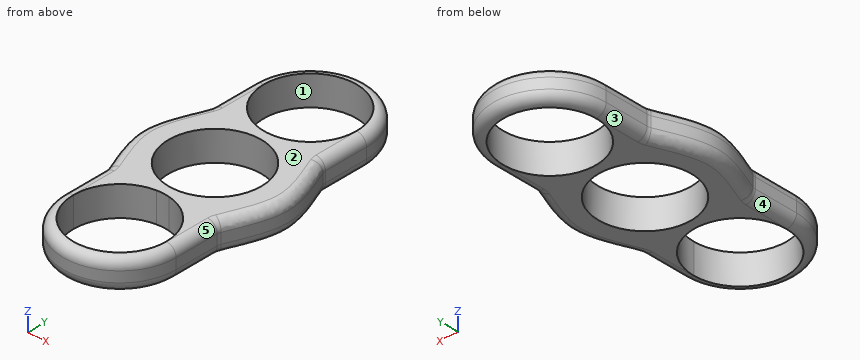
```python
from build123d import *

# Parameters (mm, degrees)
F0_R     = 11.1
F1_DEPTH = 7.1
F2_R     = 2.3


with BuildPart() as f1:
    # F0 (on Top) → F1 (new body)
    with BuildSketch(Plane.XY):
        with BuildLine():
            Line((11.1, 24.4949632536), (13.5, 24.4949632536))
            ThreePointArc((13.5, 24.4949632536), (0, 37.9949632536), (-13.5, 24.4949632536))
            Line((-13.5, 24.4949632536), (-11.1, 24.4949632536))
            ThreePointArc((-11.1, 24.4949632536), (0, 35.5949632536), (11.1, 24.4949632536))
        make_face()
        with BuildLine():
            Line((-13.5, 13.5), (-1.5234116489, 13.5))
            ThreePointArc((-1.5234116489, 13.5), (-8.3701812795, 17.2045541191), (-11.1, 24.4949632536))
            Line((-11.1, 24.4949632536), (-13.5, 24.4949632536))
            Line((-13.5, 24.4949632536), (-13.5, 13.5))
        make_face()
        with BuildLine():
            Line((1.5234116489, 13.5), (13.5, 13.5))
            Line((13.5, 13.5), (13.5, 24.4949632536))
            Line((13.5, 24.4949632536), (11.1, 24.4949632536))
            ThreePointArc((11.1, 24.4949632536), (8.3701812795, 17.2045541191), (1.5234116489, 13.5))
        make_face()
        with BuildLine():
            Line((13.5, -13.5), (13.5, 13.5))
            Line((13.5, 13.5), (1.5234116489, 13.5))
            ThreePointArc((1.5234116489, 13.5), (0, 13.3949632536), (-1.5234116489, 13.5))
            Line((-1.5234116489, 13.5), (-13.5, 13.5))
            Line((-13.5, 13.5), (-13.5, -13.5))
            Line((-13.5, -13.5), (-1.5048250316, -13.5))
            ThreePointArc((-1.5048250316, -13.5), (0, -13.3975225221), (1.5048250316, -13.5))
            Line((1.5048250316, -13.5), (13.5, -13.5))
        make_face()
        Circle(F0_R, mode=Mode.SUBTRACT)
        with BuildLine():
            add(Edge.make_bspline(
                [(13.5, 13.5), (15.2430341691, 9), (19.7569658309, 0), (15.2430341691, -9), (13.5, -13.5)],
                knots=[0, 0, 0, 0, 0.5, 1, 1, 1, 1], degree=3))
            Line((13.5, 13.5), (13.5, -13.5))
        make_face()
        with BuildLine():
            Line((-13.5, -13.5), (-13.5, 13.5))
            add(Edge.make_bspline(
                [(-13.5, 13.5), (-15.2435445338, 9), (-19.7564554662, 0), (-15.2435445338, -9), (-13.5, -13.5)],
                knots=[0, 0, 0, 0, 0.5, 1, 1, 1, 1], degree=3))
        make_face()
        with BuildLine():
            ThreePointArc((-11.1, -24.4975225221), (-8.3640169133, -17.2000420614), (-1.5048250316, -13.5))
            Line((-1.5048250316, -13.5), (-13.5, -13.5))
            Line((-13.5, -13.5), (-13.5, -24.4975225221))
            Line((-13.5, -24.4975225221), (-11.1, -24.4975225221))
        make_face()
        with BuildLine():
            Line((13.5, -24.4975225221), (13.5, -13.5))
            Line((13.5, -13.5), (1.5048250316, -13.5))
            ThreePointArc((1.5048250316, -13.5), (8.3640169133, -17.2000420614), (11.1, -24.4975225221))
            Line((11.1, -24.4975225221), (13.5, -24.4975225221))
        make_face()
        with BuildLine():
            ThreePointArc((-13.5, -24.4975225221), (0, -37.9975225221), (13.5, -24.4975225221))
            Line((13.5, -24.4975225221), (11.1, -24.4975225221))
            ThreePointArc((11.1, -24.4975225221), (0, -35.5975225221), (-11.1, -24.4975225221))
            Line((-11.1, -24.4975225221), (-13.5, -24.4975225221))
        make_face()
    extrude(amount=F1_DEPTH)

    # F2
    f2_edges = [f1.edges().sort_by_distance(p)[0] for p in [
        (13.5, -13.5, 3.55),
        (17.5, 0, 7.1),
        (17.5, 0, 0),
        (13.5, 13.5, 3.55),
        (13.5, 18.997482, 7.1),
        (0, 37.994963, 7.1),
        (0, 37.994963, 0),
        (13.5, 24.494963, 3.55),
        (13.5, 18.997482, 0),
        (-13.5, 18.997482, 7.1),
        (-17.5, 0, 7.1),
        (0, -37.997523, 7.1),
        (-13.5, -18.998761, 7.1),
        (13.5, -18.998761, 7.1),
        (13.5, -18.998761, 0),
        (0, -37.997523, 0),
        (-13.5, -13.5, 3.55),
        (-13.5, 13.5, 3.55),
        (-13.5, 18.997482, 0),
        (-17.5, 0, 0),
        (-13.5, -18.998761, 0),
    ]]
    fillet(f2_edges, radius=F2_R)


solid = f1.part
```
For this review, take the finished solid that the model builds, in its own axes (mm). Face numbers are marked on the shaded views. A direction names the side the tool comes from. Coordinates: 2 decimals unless noted, no trailing zeros. Loops run counter-clockwise (first coordinate to the right, second up) from the corner with the lowest first, then second, coordinate; pieces in that order, holes last.
1. For line 1 (Y direction, x = -5, z = 6); line 2 (Y direction, x = -5.5, z = 3.5); line 3 (X direction, y = -26, z = 1.75), list the stretches that pass through material, from the lowest coordinate up.
2. Add section B-B, the plane y = 16. Give the boundary of the cut face in (x, z), then the cut area to 3 significant figures.
3. Add section C-C, the plane x = 5. Count the separate pieces of the cut face and the enclosed holes in it, then the cut area to 3 significant figures.
4. Insertion check: P1, Ø3, axis at x = 4, z = 6, coming from the -Y side; P2, Ø0.8, axis at y = -20, z = 3.5, coming from the -X side; P3, Ø1, axis at y = -10.5, z = 3.5, coming from the -X side; P4, Ø1.5, axis at x = -8, y = 13, coming from the -Z side. Each pin has a flat end and moves straight along its axis. Give the tip position at first contact, or say it passes through.
5. Add section A-A, the plane x = 0. Give the boundary of the cut face in (y, z), then the cut area to 3 significant figures.
6. For the marked faces 3, 4 and 5, list the 3-axis set-ups (+Z, -Z, +X, -X, +Y, -Y) from which the entire face can be reached by the end or side of a thin tool; tool diameter is ignored.
7. Mouldability with a two-part tool opening along Y and no side actions: class the marked faces 1 and 2 as +Y half, -Y half, draft (parallel to the pull), parting line (faces both ways), or undercut.
Result:
1. line 1: y = -36.67 to -34.41, -14.59 to -9.91, 9.91 to 14.58, 34.41 to 36.67
1. line 2: y = -36.83 to -34.14, -14.86 to -9.64, 9.64 to 14.85, 34.14 to 36.82
1. line 3: x = -13.35 to -11, 11 to 13.35
2. outline: (-13.5, 2.3) arc R2.3 ccw to (-11.2, 0) - (-7.14, 0) - (-7.14, 7.1) - (-11.2, 7.1) arc R2.3 ccw to (-13.5, 4.8) - close; (7.14, 0) - (11.2, 0) arc R2.3 ccw to (13.5, 2.3) - (13.5, 4.8) arc R2.3 ccw to (11.2, 7.1) - (7.14, 7.1) - close
2. area: 85.7 mm2
3. separate pieces: 4
3. enclosed holes: 0
3. area: 98.8 mm2
4. P1: stops at y = -37.68
4. P2: stops at x = -13.5
4. P3: stops at x = -14.91
4. P4: stops at z = 0
5. outline: (-38, 2.3) arc R2.3 ccw to (-35.7, 0) - (-35.6, 0) - (-35.6, 7.1) - (-35.7, 7.1) arc R2.3 ccw to (-38, 4.8) - close; (-13.4, 0) - (-11.1, 0) - (-11.1, 7.1) - (-13.4, 7.1) - close; (11.1, 0) - (13.39, 0) - (13.39, 7.1) - (11.1, 7.1) - close; (35.59, 0) - (35.69, 0) arc R2.3 ccw to (37.99, 2.3) - (37.99, 4.8) arc R2.3 ccw to (35.69, 7.1) - (35.59, 7.1) - close
5. area: 62.1 mm2
6. face 3: -Z, -X, +Y
6. face 4: -Z, -X, -Y
6. face 5: +Z, +X, -Y
7. face 1: undercut
7. face 2: draft
